Geometry check sheet. Reference: the model listing, model coordinates, mm. Round coordinates to 2 decimals unless told otherwise and drop trailing zeros. Write each loop counter-clockwise with the first axis right and the second up, starting at its lowest first coordinate (ties: lowest second). Pieces come first, ordered by that corner, then holes. Notation, with made-up numbers: M -20.75,45 L 21.25,45 A20 cw 21.25,53 Z; hole C 5.5,-33.75 d5. An arc over 180 degrees is marked long. Answer as CSV lines item,"result". Start each with the question number.
```python
from build123d import *

# Parameters (mm, degrees)
F0_R     = 216.451493
F0_R_2   = 150
F1_DEPTH = 3
F2_R     = 5
F3_DEPTH = 3
F4_R     = 2.5
F5_DEPTH = 3


with BuildPart() as f1:
    # F0 (on Top) → F1 (new body)
    with BuildSketch(Plane.XY):
        Circle(F0_R)
        Circle(F0_R_2, mode=Mode.SUBTRACT)
    extrude(amount=F1_DEPTH)

    # F2 (on face) → F3 (cut)
    with BuildSketch(Plane.XY.offset(3)):
        with BuildLine():
            ThreePointArc((0, 195), (3.535534, 196.464466), (5, 200))
            ThreePointArc((5, 200), (-3.535534, 203.535534), (0, 195))
        make_face()
        with Locations((-173.205081, -100)):
            Circle(F2_R)
        with Locations((173.205081, -100)):
            Circle(F2_R)
    extrude(amount=-F3_DEPTH, mode=Mode.SUBTRACT)

    # F4 (on face) → F5 (cut)
    with BuildSketch(Plane.XY.offset(3)):
        with BuildLine():
            ThreePointArc((0, 154.5), (1.767767, 155.232233), (2.5, 157))
            ThreePointArc((2.5, 157), (-1.767767, 158.767767), (0, 154.5))
        make_face()
        with Locations((-157, 0)):
            Circle(F4_R)
        with Locations((0, -157)):
            Circle(F4_R)
        with Locations((157, 0)):
            Circle(F4_R)
    extrude(amount=-F5_DEPTH, mode=Mode.SUBTRACT)


solid = f1.part
```
1) Scan lines: line 1 (Y direction, x = 0, z = 1.1); line 2 (X direction, y = 122.5, z = 1.4); line 3 (X direction, y = 60, z = 1.1). Record each from-to range of solid material in increasing order. Write a range as from..to.
2) Section check A-A, the plane x = -141. Record the cut outline in (y, z).
3) Mould release check, pull along X, two halves, no side actions. Record for faces 1 (the cylindrical face through (-46.922, -211.304, 1.479)), 2 (the flat face through (-51.1, -141.3, 0)), 3 (the cylindrical face through (-178.2, -99.8, 1.5)): released by +X, released by -X, zero draft, split by the parting line, or undercut.
4) Section check C-C, the plane z = 2.1. Give the number of separate pieces and of enclosed holes in the cut face, plus the area to 3 significant figures.
5) Go/stop test with flat-tipped pins: pin 1 (8 mm diameter, centred on x = 157, y = 0, fed in from +Z); pin 2 (8 mm diameter, centred on x = -173.21, y = -100, fed in from -Z); pin 3 (1.5 mm diameter, centred on x = 76, z = 1, fed in from +Y). Record where each tip stops, or that it passes through.
6) Section check D-D, the plane y = -100. Record the cut outline in (x, z), plus the area to 3 significant figures.
7) Section check B-B, the plane y = 69. Record the cut outline in (x, z).
Results:
1,line 1,"y = -216.45..-159.5, -154.5..-150, 150..154.5, 159.5..195, 205..216.45"
1,line 2,"x = -178.45..-86.57, 86.57..178.45"
1,line 3,"x = -207.97..-137.48, 137.48..207.97"
2,outline,"M -164.23,0 L -51.18,0 L -51.18,3 L -164.23,3 Z; M 51.18,0 L 164.23,0 L 164.23,3 L 51.18,3 Z"
3,face 1,"split by the parting line"
3,face 2,"zero draft"
3,face 3,"undercut"
4,separate pieces,"1"
4,enclosed holes,"8"
4,area,"76,200 mm^2"
5,pin 1,"stops at z = 3"
5,pin 2,"passes through"
5,pin 3,"stops at y = 202.95"
6,outline,"M -191.97,0 L -178.21,0 L -178.21,3 L -191.97,3 Z; M -168.21,0 L -111.8,0 L -111.8,3 L -168.21,3 Z; M 111.8,0 L 168.21,0 L 168.21,3 L 111.8,3 Z; M 178.21,0 L 191.97,0 L 191.97,3 L 178.21,3 Z"
6,area,"421 mm^2"
7,outline,"M -205.16,0 L -133.19,0 L -133.19,3 L -205.16,3 Z; M 133.19,0 L 205.16,0 L 205.16,3 L 133.19,3 Z"
